Geometry: final body of the model. Coordinates: model frame, mm. Coordinates: 2 decimals unless noted, no trailing zeros. Loops run counter-clockwise (first coordinate to the right, second up) from the corner with the lowest first, then second, coordinate; pieces in that order, holes last. Notation, with made-up numbers: (23, -22) -> (38, -22) arc R18 cw to (38, 6) -> close; hole circle Ø2 at (80.25, -18). An arc over 180 degrees is marked (long way). One line per item, written item: value. Start each with the question number.
Item 1: Ray query, probe 1 along Y at (x, z) = (4.75, 246.5); probe 2 along Y at (x, z) = (4.5, 66); probe 3 along X at (y, z) = (-2.15, 212.5). Return the intervals inside material, ascending. Write a range as from..to.
Item 2: Section query B-B on z = 29.5. Return loops of the section in (x, y) (3 decimals), then the cut area to 3 significant figures.
Item 3: Mould query, pull axis Z, two halves, no side actions, for faces 1 (the flat face through (0, 0, 300)), 2 (the flat face through (2, -0.5, 212)). Classes: +Z half, -Z half, draft (parallel to the pull), parting line (faces both ways), or undercut.
Item 4: Section query A-A on y = -2.25. Give the number of separate pieces and of enclosed holes in the cut face, then the cut area to 3 significant figures.
Item 5: Contact query for a flat-ended pin moving along its axis: pin 1 Ø3 at (x, z) = (-1, 212.5) entering from +Y. Output: stop coordinate, or through.
from build123d import *

# Parameters (mm, degrees)
BOSS_EXTRUDE1_DEPTH = 300
SKETCH2_R           = 3
CUT_EXTRUDE1_DEPTH  = 4.5
SKETCH3_R           = 1.75
CUT_EXTRUDE2_DEPTH  = 4.5
LPATTERN1_COUNT     = 14
LPATTERN1_PITCH     = 25


with BuildPart() as part:
    # Sketch1 → Boss-Extrude1 (new body)
    with BuildSketch(Plane.XY):
        with BuildLine():
            Line((6, -3.5), (6, 0.368911094))
            ThreePointArc((6, 0.368911094), (5.63354293, 0.61854293), (5.383911094, 0.985))
            Line((5.383911094, 0.985), (4.92112495, 0.985))
            ThreePointArc((4.92112495, 0.985), (4.265, 1.46), (4.92112495, 1.935))
            Line((4.92112495, 1.935), (5.383911094, 1.935))
            ThreePointArc((5.383911094, 1.935), (5.63354293, 2.30145707), (6, 2.551088906))
            Line((6, 2.551088906), (6, 3.5))
            Line((6, 3.5), (5.5, 4))
            Line((5.5, 4), (-5.5, 4))
            Line((-5.5, 4), (-6, 3.5))
            Line((-6, 3.5), (-6, 2.551088906))
            ThreePointArc((-6, 2.551088906), (-5.63354293, 2.30145707), (-5.383911094, 1.935))
            Line((-5.383911094, 1.935), (-4.92112495, 1.935))
            ThreePointArc((-4.92112495, 1.935), (-4.265, 1.46), (-4.92112495, 0.985))
            Line((-4.92112495, 0.985), (-5.383911094, 0.985))
            ThreePointArc((-5.383911094, 0.985), (-5.63354293, 0.61854293), (-6, 0.368911094))
            Line((-6, 0.368911094), (-6, -3.5))
            Line((-6, -3.5), (-5.5, -4))
            Line((-5.5, -4), (5.5, -4))
            Line((5.5, -4), (6, -3.5))
        make_face()
    extrude(amount=BOSS_EXTRUDE1_DEPTH)

    # Sketch2 → Cut-Extrude1 (cut)
    with BuildSketch(Plane(origin=(0, 4, 0), x_dir=(1, 0, 0), z_dir=(0, 1, 0))):
        with Locations((0, -12.5)):
            Circle(SKETCH2_R)
    cut_extrude1 = extrude(amount=-CUT_EXTRUDE1_DEPTH, mode=Mode.SUBTRACT)

    # Sketch3 → Cut-Extrude2 (cut, through all)
    with BuildSketch(Plane(origin=(0, -0.5, 0), x_dir=(1, 0, 0), z_dir=(0, 1, 0))):
        with Locations((0, -12.5)):
            Circle(SKETCH3_R)
    cut_extrude2 = extrude(amount=-CUT_EXTRUDE2_DEPTH, mode=Mode.SUBTRACT)

    # LPattern1: Cut-Extrude1, Cut-Extrude2 ×14
    with Locations(*[(0, 0, i * LPATTERN1_PITCH) for i in range(1, LPATTERN1_COUNT)]):
        add(cut_extrude1, mode=Mode.SUBTRACT)
        add(cut_extrude2, mode=Mode.SUBTRACT)


solid = part.part
Reply:
1. probe 1: y = -4..0.96, 1.96..4
1. probe 2: y = -4..1.04, 1.88..4
1. probe 3: x = -6..-1.75, 1.75..6
2. outline: (-6, -3.5) -> (-5.5, -4) -> (5.5, -4) -> (6, -3.5) -> (6, 0.369) arc R1.19 cw to (5.384, 0.985) -> (4.921, 0.985) arc R0.5 cw (long way) to (4.921, 1.935) -> (5.384, 1.935) arc R1.19 cw to (6, 2.551) -> (6, 3.5) -> (5.5, 4) -> (-5.5, 4) -> (-6, 3.5) -> (-6, 2.551) arc R1.19 cw to (-5.384, 1.935) -> (-4.921, 1.935) arc R0.5 cw (long way) to (-4.921, 0.985) -> (-5.384, 0.985) arc R1.19 cw to (-6, 0.369) -> close
2. area: 91.4 mm²
3. face 1: +Z half
3. face 2: undercut
4. separate pieces: 1
4. enclosed holes: 12
4. area: 3,480 mm²
5. pin 1: stops at y = -0.5
